Work out the finished part from the listing and answer in its coordinate system (mm). A direction names the side the tool comes from. Coordinates: 2 decimals unless noted, no trailing zeros. Order: outer loops, then holes, each group sorted by start corner. A loop starts at its lowest first (then second) coordinate and runs counter-clockwise, first axis right, second up.
1. The part is cut by section C-C, the plane x = -2.25. Give the vertices of the cut face in (y, z), then the cut area to 3 significant figures.
2. A tool of negligible diameter and unlimited length cuts with its end or side. For faces 1 (the flat face through (-1, -11.112, 9)), 2 (the flat face through (12.7, 0, 9)), from which of +Z, -Z, +X, -X, +Y, -Y can it reach the whole face along a straight path? Write none if from no direction.
3. The part is cut by section B-B, the plane y = -2.75. Give the vertices of the cut face in (x, z).
4. The part is cut by section A-A, the plane z = -524.5. Give the vertices of the cut face in (x, y).
5. Flat-ended cylindrical pins translate along their axes: pin 1 Ø12 at (x, y) = (6.5, -3.5) entering from +Z; pin 2 Ø10.5 at (y, z) = (4, 48.5) entering from -X. Find the tip coordinate at first contact, or state that the pin passes through.
6. Find the intervals of material crossed by probe 1 along X at (y, z) = (-1, 288); probe 2 along Y at (x, z) = (-11.5, 428.5); probe 3 along X at (y, z) = (-10.75, 114), in increasing order.
```python
from build123d import *

# Parameters (mm, degrees)
BOSS_EXTRUDE1_DEPTH = 609.6


with BuildPart() as part:
    # Sketch2 → Boss-Extrude1 (new, symmetric)
    with BuildSketch(Plane.XY):
        with BuildLine():
            Line((-12.7, -12.7), (12.7, -12.7))
            Line((12.7, -12.7), (12.7, 12.7))
            Line((12.7, 12.7), (11.90625, 12.7))
            ThreePointArc((11.90625, 12.7), (11.344983992, 12.467516008), (11.1125, 11.90625))
            Line((11.1125, 11.90625), (11.1125, -9.5377))
            ThreePointArc((11.1125, -9.5377), (10.651251759, -10.651251759), (9.5377, -11.1125))
            Line((9.5377, -11.1125), (-11.90625, -11.1125))
            ThreePointArc((-11.90625, -11.1125), (-12.467516008, -11.344983992), (-12.7, -11.90625))
            Line((-12.7, -11.90625), (-12.7, -12.7))
        make_face()
    extrude(amount=BOSS_EXTRUDE1_DEPTH, both=True)


solid = part.part
```
Geometry says:
1. outline: (-12.7, -609.6) - (-11.11, -609.6) - (-11.11, 609.6) - (-12.7, 609.6) - close
1. area: 1,940 mm2
2. face 1: +Z, -Z, -X, +Y
2. face 2: +Z, -Z, +X, +Y, -Y
3. outline: (11.11, -609.6) - (12.7, -609.6) - (12.7, 609.6) - (11.11, 609.6) - close
4. outline: (-12.7, -12.7) - (12.7, -12.7) - (12.7, 12.7) - (11.91, 12.7) arc R0.79 ccw to (11.11, 11.91) - (11.11, -9.54) arc R1.57 cw to (9.54, -11.11) - (-11.91, -11.11) arc R0.79 ccw to (-12.7, -11.91) - close
5. pin 1: stops at z = 609.6
5. pin 2: stops at x = 11.11
6. probe 1: x = 11.11 to 12.7
6. probe 2: y = -12.7 to -11.11
6. probe 3: x = 10.54 to 12.7
